Input: part model. Units: mm. Frame: model coordinates. Face numbers are marked on the shaded views. Coordinates: 2 decimals unless noted, no trailing zeros. Write each loop counter-clockwise with the first axis right and the second up, starting at its lowest first coordinate (ties: lowest second). Pieces come first, ordered by that corner, then holes. Notation, with made-up numbers: (89.5, -25.5) - (143.5, -25.5) arc R21 ccw to (143.5, 13.5) - close; hole circle Ø5 at (-21.5, -11.5). An arc over 180 degrees is marked (long way). Put each result on its own line as item: value. Start each with the question number.
1. Line query: line 1 (Y direction, x = 0, z = -0.75). Output: solid intervals per line, ascending.
2. Cut plane A-A, the plane y = 0. Return loops of the section in (x, z).
3. Pull-direction query (Z, two-part tool) for the marked faces 1, 2 and 3; classes: released by +Z, released by -Z, zero draft, split by the parting line, or undercut.
4. Cut plane B-B, the plane x = -10. Count the separate pieces of the cut face and the enclosed holes in it, and give its area (3 significant figures).
5. Pin query (flat end, axial travel): pin 1 (1.5 mm diameter, centred on x = 0, z = 0, fed in from +Y); pin 2 (2 mm diameter, centred on x = -12.5, z = 0, fed in from -Y); pin 3 (1.5 mm diameter, centred on x = -5.5, z = 2.5, fed in from -Y). Return the tip coordinate at first contact, or that it passes through.
Autodesk Inventor part; units mm, degrees
ref_plane "Work Plane2" through (0, 17, 0) normal (0, 1, 0) x (-1, 0, 0)
ref_plane "Work Plane3" through (14.7224, -8.5, 0) normal (0.866, -0.5, 0) x (0.5, 0.866, 0)
ref_plane "Work Plane4" through (-14.7224, -8.5, 0) normal (-0.866, -0.5, 0) x (0.5, -0.866, 0)
sketch "Sketch2" plane through (0, 0, 0) normal (0, 0, 1) x (1, 0, 0)
  circle A0 centre (0, 0) radius 17
  dimension "d0" = 34
extrude "Extrusion1" add sketch "Sketch2" along normal mid plane 7
ref_plane "Work Plane2" through (0, 17, 0) normal (0, 1, 0) x (-1, 0, 0)
sketch "Sketch3" plane through (0, 17, 0) normal (0, 1, 0) x (-1, 0, 0)
  point P0 (0, 0)
  point P1 (0, 0)
sketch "Sketch4" plane through (0, 0, 0) normal (0, 0, 1) x (1, 0, 0)
  circle A0 centre (0, 0) radius 17
  point P0 (0, 17)
  point P1 (0, 17)
  point P2 (0, 17)
  point P3 (-14.7224, -8.5)
  point P4 (-14.7224, -8.5)
  point P5 (-14.7224, -8.5)
  point P6 (14.7224, -8.5)
  point P7 (14.7224, -8.5)
  point P8 (14.7224, -8.5)
  dimension "d5" = 360
ref_plane "Work Plane3" through (14.7224, -8.5, 0) normal (0.866, -0.5, 0) x (0.5, 0.866, 0)
ref_plane "Work Plane4" through (-14.7224, -8.5, 0) normal (-0.866, -0.5, 0) x (0.5, -0.866, 0)
sketch "Sketch5" plane through (-14.7224, -8.5, 0) normal (-0.866, -0.5, 0) x (0.5, -0.866, 0)
  point P0 (0, 0)
ref_plane "Work Plane5" through (0, 0, 0) normal (0, 0, 1) x (1, 0, 0)
sketch "Sketch8" plane through (0, 0, 3.5) normal (0, 0, 1) x (1, 0, 0)
  circle A0 centre (0, 0) radius 12
  point P0 (0, -12)
  point P1 (10.3923, 6)
  point P2 (-10.3923, 6)
  dimension "d7" = 24
  dimension "d10" = 360
sketch "Sketch9" plane through (0, 0, 0) normal (0, 0, 1) x (1, 0, 0)
  point P0 (0, 0)
hole "Hole3" at (0, 0, 3.5) direction (0, 0, -1) diameter 3.242 end through all
sketch "Sketch12" plane through (0, 17, 0) normal (0, 1, 0) x (-1, 0, 0)
  point P0 (0, 0)
sketch "Sketch13" plane through (0, 17, 0) normal (0, 1, 0) x (-1, 0, 0)
  point P0 (0, 0)
  point P1 (0, 0)
hole "Hole4" at (0, 17, 0) direction (0, -1, 0) diameter 2.459 depth 8.8 tip angle 118
pattern_circular "Circular Pattern1" count 3 over 360 about axis through (0, 0, -10) along (0, 0, 1) of "Hole4"
chamfer "Chamfer1" distance 0.3 angle 45 10 edges at (0, 1.621, -3.5) (0, 1.621, 3.5) (0.922, 16.975, 0.8134) (0.9217, 16.975, -0.8138) (-0.9219, 16.975, 0.8135) (-0.9217, 16.975, -0.8138) (15.2986, -7.413, -0.0002) (14.0691, -9.5425, 0.002) (-14.0691, -9.5425, -0.0002) (-15.2986, -7.413, 0.002)
chamfer "Chamfer2" distance 0.5 angle 45 2 edges at (-17, 0, 3.5) (-17, 0, -3.5)
sketch "Sketch14" plane through (0, 0, -3.5) normal (0, 0, -1) x (-1, 0, 0)
  point P0 (0, 0)
  point P1 (0, -12)
  point P2 (10.3923, 6)
  point P3 (-10.3923, 6)
  dimension "d42" = 12
  dimension "d45" = 360
hole "Hole5" at (-10.3923, 6, -3.5) at (10.3923, 6, -3.5) at (0, -12, -3.5) direction (0, 0, 1) diameter 3.4 end through all countersink diameter 6.3 countersink angle 90
sketch "Sketch10" plane through (0, 0, 3.5) normal (0, 0, 1) x (1, 0, 0)
  point P0 (10.3923, 6)
  point P1 (0, -12)
  point P2 (-10.3923, 6)
properties part number "srodek_pajaka" material "Aluminum 6061"
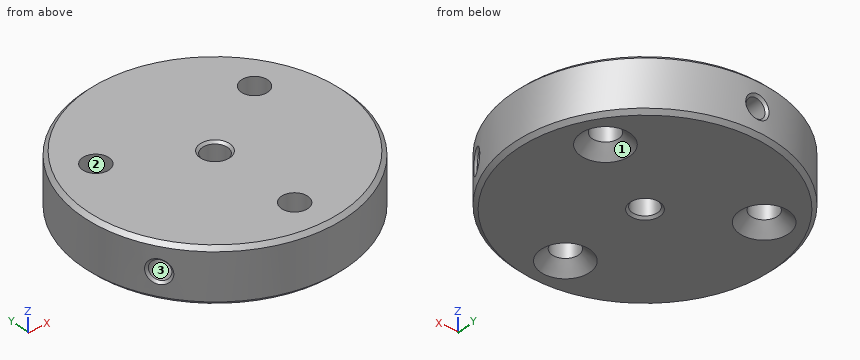
Report:
1. line 1: y = -17 to -13.7, -10.3 to -1.62, 1.62 to 7.91
2. outline: (-17, -3) - (-16.5, -3.5) - (-1.92, -3.5) - (-1.62, -3.2) - (-1.62, 3.2) - (-1.92, 3.5) - (-16.5, 3.5) - (-17, 3) - close; (1.62, -3.2) - (1.92, -3.5) - (16.5, -3.5) - (17, -3) - (17, 3) - (16.5, 3.5) - (1.92, 3.5) - (1.62, 3.2) - close
3. face 1: released by -Z
3. face 2: zero draft
3. face 3: undercut
4. separate pieces: 2
4. enclosed holes: 1
4. area: 161 mm^2
5. pin 1: stops at y = 7.91
5. pin 2: stops at y = -12.52
5. pin 3: stops at y = -16.32
